```python
from build123d import *

# Parameters (mm, degrees)
SKETCH2_R          = 1.25
CUT_EXTRUDE1_DEPTH = 10


with BuildPart() as part:
    # Sketch1 → Revolve1 (revolve)
    with BuildSketch(Plane.XY, mode=Mode.PRIVATE) as revolve1_sk:
        Polygon((11, 0), (11, 14), (15, 14), (15, 6), (22, 6), (22, 0), align=None)
    revolve(revolve1_sk.sketch.rotate(Axis((0, 0, 0), (0, 1, 0)), 90), axis=Axis((0, 0, 0), (0, 1, 0)))

    # Sketch2 → Cut-Extrude1 (cut)
    with BuildSketch(Plane(origin=(0, 6, 0), x_dir=(1, 0, 0), z_dir=(0, 1, 0))):
        with Locations(Location((0, 18.5, 0), (0, 0, 270))):
            Circle(SKETCH2_R)
        with Locations(Location((16.02146997, 9.25, 0), (0, 0, 270))):
            Circle(SKETCH2_R)
        with Locations(Location((16.02146997, -9.25, 0), (0, 0, 270))):
            Circle(SKETCH2_R)
        with Locations(Location((0, -18.5, 0), (0, 0, 270))):
            Circle(SKETCH2_R)
        with Locations(Location((-16.02146997, -9.25, 0), (0, 0, 270))):
            Circle(SKETCH2_R)
        with Locations(Location((-16.02146997, 9.25, 0), (0, 0, 270))):
            Circle(SKETCH2_R)
    extrude(amount=-CUT_EXTRUDE1_DEPTH, mode=Mode.SUBTRACT)


solid = part.part
```
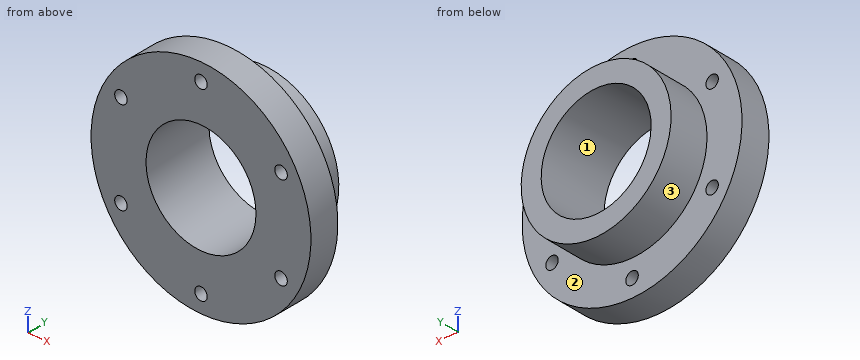
Could you check a few things on this model? Use its own coordinates, in mm. Face numbers are marked on the shaded views. Round coordinates to 2 decimals unless told otherwise and drop trailing zeros. Write each loop counter-clockwise with the first axis right and the second up, starting at its lowest first coordinate (ties: lowest second). Pieces come first, ordered by that corner, then holes. Notation, with made-up numbers: M -7.5,62.25 L 47.5,62.25 A24 ccw 47.5,85.25 Z; hole C 60.5,78 d9. An arc over 180 degrees is marked long. Write each question's results on one line, items separated by ' | '. Start each with the question number.
1. I need wall thicknesses on L1, parallel to X at y = 2, z = 10; L2, parallel to X at y = 4.5, z = 0; L3, parallel to X at y = 2.35, z = 9.25. Which ranges of each line are inside material? Lowest first, please. Write a range as from..to.
2. Imagine slicing it at B-B on x = -5. List the corners of the cut face in (y, z) for me.
3. Imagine slicing it at C-C on z = 18.5. List the corners of the cut face in (x, y) for me.
4. Thinking about a two-plate mould opening in X: for the marked faces 1, 2 and 3, which applies, +X half, -X half, draft (parallel to the pull), parting line (faces both ways), or undercut?
5. Imagine slicing it at D-D on z = 9. List the corners of the cut face in (x, y) for me, and give its area (3 significant figures).
6. I'm going to push flat-ended pins straight in: pin 1 Ø4 at (x, y) = (12, 7) entering from +Z; pin 2 Ø3 at (y, z) = (2, -15.5) entering from -X; pin 3 Ø3 at (y, z) = (12.5, -7) entering from -X. Where does each tip first touch, or does it pass through?
7. Imagine slicing it at A-A on x = 0. List the corners of the cut face in (y, z) for me, and give its area (3 significant figures).
Result sheet:
1) L1: x = -19.6..-17.02, -15.02..-4.58, 4.58..15.02, 17.02..19.6 | L2: x = -22..-11, 11..22 | L3: x = -19.96..-17.27, -14.77..-5.95, 5.95..14.77, 17.27..19.96
2) outline: M 0,-21.42 L 6,-21.42 L 6,-14.14 L 14,-14.14 L 14,-9.8 L 0,-9.8 Z; M 0,9.8 L 14,9.8 L 14,14.14 L 6,14.14 L 6,21.42 L 0,21.42 Z
3) outline: M -11.91,0 L -1.25,0 L -1.25,6 L -11.91,6 Z; M 1.25,0 L 11.91,0 L 11.91,6 L 1.25,6 Z
4) face 1: undercut | face 2: draft | face 3: parting line
5) outline: M -20.07,0 L -17.25,0 L -17.25,6 L -20.07,6 Z; M -14.8,0 L -6.32,0 L -6.32,14 L -12,14 L -12,6 L -14.8,6 Z; M 6.32,0 L 14.8,0 L 14.8,6 L 12,6 L 12,14 L 6.32,14 Z; M 17.25,0 L 20.07,0 L 20.07,6 L 17.25,6 Z | area: 226 mm^2
6) pin 1: stops at z = 19.46 | pin 2: stops at x = -16.97 | pin 3: stops at x = -13.96
7) outline: M 0,-22 L 6,-22 L 6,-19.75 L 0,-19.75 Z; M 0,-17.25 L 6,-17.25 L 6,-15 L 14,-15 L 14,-11 L 0,-11 Z; M 0,11 L 14,11 L 14,15 L 6,15 L 6,17.25 L 0,17.25 Z; M 0,19.75 L 6,19.75 L 6,22 L 0,22 Z | area: 166 mm^2
